Design review of the part built by this model. Coordinates are the model's own, in mm. Face numbers are marked on the shaded views. A direction names the side the tool comes from. Give positions to 0.01 mm unless a question says otherwise; leave off trailing zeros. Write each loop counter-clockwise with the first axis right and the second up, starting at its lowest first coordinate (ties: lowest second). Pieces come first, ordered by that corner, then holes. Notation, with made-up numbers: (69, -6) -> (80, -6) arc R13 cw to (80, 19) -> close; hole circle Ø10 at (-18.5, 25). An arc over 180 degrees is marked (long way). Answer as a JSON object with one key per item and string values.
Autodesk Fusion 360 part; units mm, degrees
sketch "Sketch1" plane through (0, 0, 0) normal (0, 0, 1) x (1, 0, 0)
  line L0 (21, -21) -> (-21, -21)
  line L1 (-21, -21) -> (-21, 21)
  line L2 (-21, 21) -> (21, 21)
  line L3 (21, 21) -> (21, -21)
  line L4 (21, -21) -> (-21, 21) construction
  line L5 (-21, -21) -> (21, 21) construction
  line L6 (0, 50) -> (0, -40)
  line L7 (-140, 50) -> (140, 50)
  line L8 (140, 50) -> (140, -130)
  line L9 (140, -130) -> (-140, -130)
  line L10 (-140, -130) -> (-140, 50)
  line L11 (-140, 50) -> (140, -130) construction
  line L12 (140, 50) -> (-140, -130) construction
  point P0 (0, -40)
  dimension "d1" = 42
  dimension "d2" = 42
  dimension "d14" = 280
extrude "Extrude4" add sketch "Sketch1" along normal blind 10
sketch "Sketch3" plane through (0, 0, 10) normal (0, 0, 1) x (-1, 0, 0)
  line L0 (21, -21) -> (-21, -21)
  line L1 (-21, -21) -> (-21, 21)
  line L2 (-21, 21) -> (21, 21)
  line L3 (21, 21) -> (21, -21)
  line L4 (140, 130) -> (-140, 130)
  line L5 (-140, 130) -> (-140, -50)
  line L6 (-140, -50) -> (140, -50)
  line L7 (140, -50) -> (140, 130)
  line L8 (-120, 120) -> (40, 120)
  line L9 (40, 120) -> (40, 35)
  line L10 (40, 35) -> (-120, 35)
  line L11 (-120, 35) -> (-120, 120)
  line L12 (70, 100) -> (126, 100)
  line L13 (126, 100) -> (126, 15)
  line L14 (126, 15) -> (70, 15)
  line L15 (70, 15) -> (70, 100)
  line L16 (-140, -50) -> (-135, -50)
  line L17 (-135, -50) -> (-135, 130)
  line L18 (-135, 130) -> (-140, 130)
  line L19 (-140, 130) -> (-140, -50)
  line L20 (-135, 130) -> (140, 130)
  line L21 (140, 130) -> (140, 125)
  line L22 (140, 125) -> (-135, 125)
  line L23 (-135, 125) -> (-135, 130)
  line L24 (140, 125) -> (135, 125)
  line L25 (135, 125) -> (135, -25)
  line L26 (135, -25) -> (140, -25)
  line L27 (140, -25) -> (140, 125)
  line L28 (135, -25) -> (25, -25)
  line L29 (25, -25) -> (25, -20)
  line L30 (25, -20) -> (135, -20)
  line L31 (135, -20) -> (135, -25)
  line L32 (25, -25) -> (-25, -25)
  line L33 (-25, -25) -> (-25, 25)
  line L34 (-25, 25) -> (25, 25)
  line L35 (25, 25) -> (25, -25)
  line L36 (25, -25) -> (-25, 25) construction
  line L37 (-25, -25) -> (25, 25) construction
  line L38 (-25, -25) -> (-135, -25)
  line L39 (-25, -21) -> (-135, -21)
  dimension "d17" = 160
  dimension "d18" = 85
  dimension "d19" = 56
  dimension "d20" = 85
  dimension "d24" = 5
  dimension "d25" = 5
  dimension "d26" = 5
  dimension "d29" = 50
  dimension "d30" = 50
extrude "Extrude6" add sketch "Sketch3" along normal blind 10 contours L4 L7 L17 L20 L21 L22 L23 L24 | L4 L5 L6 L16 L17 L18 L19 L23 | L7 L22 L24 L25 L26 L27 L31 | L25 L28 L29 L30 L31 L35
extrude "Extrude7" add sketch "Sketch3" along normal blind 10 contours L29 L32 L33 L34 L35
extrude "Extrude8" add sketch "Sketch3" along normal blind 10 contours L17 L33 L38 L39
sketch "Sketch4" plane through (0, 50, 0) normal (0, 1, 0) x (-1, 0, 0)
  line L0 (-140, 0) -> (140, 0)
  line L1 (140, 0) -> (140, 10)
  line L2 (140, 10) -> (-135, 10)
  line L3 (-135, 10) -> (-135, 20)
  line L4 (-135, 20) -> (-140, 20)
  line L5 (-140, 20) -> (-140, 0)
  line L6 (-140, 10) -> (-135, 10)
extrude "Extrude9" cut sketch "Sketch4" against normal blind 25 contours L3 L4 L5 L6
extrude "Extrude10" add 1 faces at (45, -128.3333, 20) along direction (0, 0, 1) blind 10
sketch "Sketch6" plane through (0, 0, 10) normal (0, 0, 1) x (-1, 0, 0)
  line L0 (-135, -21) -> (-25, -21)
  line L1 (-25, -21) -> (-25, 25)
  line L2 (-25, 25) -> (25, 25)
  line L3 (25, 25) -> (25, -20)
  line L4 (25, -20) -> (135, -20)
  line L5 (135, -20) -> (135, 125)
  line L6 (135, 125) -> (-135, 125)
  line L7 (-135, 125) -> (-135, -21)
  line L8 (0, 21) -> (0, 28)
  line L9 (0, 28) -> (0, 52)
  circle A0 centre (0, 28) radius 5
  circle A1 centre (0, 28) radius 7
  circle A2 centre (0, 52) radius 5
  circle A3 centre (0, 52) radius 7
  line L10 (7, 28) -> (7, 52)
  line L11 (-7, 28) -> (-7, 51)
  line L12 (5, 28) -> (5, 52)
  line L13 (-5, 28) -> (-5, 52)
  line L14 (-5, -50) -> (5, -50)
  line L15 (5, -50) -> (5, -25)
  line L16 (5, -25) -> (-5, -25)
  line L17 (-5, -25) -> (-5, -50)
  dimension "d39" = 7
  dimension "d40" = 10
  dimension "d41" = 10
  dimension "d42" = 14
extrude "Extrude11" cut sketch "Sketch6" against normal blind 20 contours L2 L8 L9 A0 | L2 L8 L9 A0 | L9 A0 A1 L13 | L9 A1 A3 L13 | L9 A0 A1 L12 | L9 A1 A3 L12 | L9 A2 A3 L13 | L9 A2 A3 L12 | A2
extrude "Extrude12" cut sketch "Sketch6" against normal blind 20 contours L14 L15 L16 L17
sketch "Sketch7" plane through (0, 21, 0) normal (0, -1, 0) x (1, 0, 0)
  line L0 (-21, 0) -> (21, 0)
  line L1 (21, 0) -> (21, 30)
  line L2 (21, 30) -> (-21, 30)
  line L3 (-21, 30) -> (-21, 0)
  line L4 (-21, 30) -> (21, 30)
  line L5 (21, 30) -> (21, 10)
  line L6 (21, 10) -> (-21, 10)
  line L7 (-21, 10) -> (-21, 30)
  dimension "d47" = 20
extrude "Extrude13" cut sketch "Sketch7" against normal blind 10 contours L1 L2 L3 L4 L5 L6 L7
extrude "Extrude14" cut 1 faces at (1.6667, 25, 3.3333) along direction (0, -1, 0) blind 5
extrude "Extrude15" add 2 faces at (50, 50, 3.3333) (-50, 50, 6.6667) along direction (0, 1, 0) blind 8
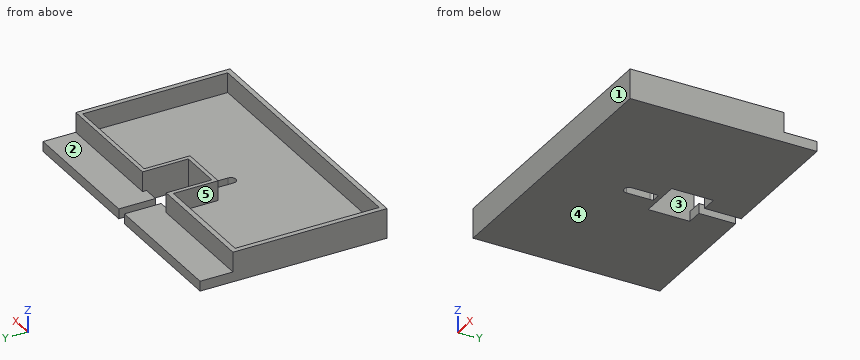
(1) For line 1 along X through (y, z) = (1.5, 19); line 2 along X through (y, z) = (-36.5, 22.25); line 3 along Y through (x, z) = (111.5, 17.5), list the stretches that pass through material, from the lowest coordinate up.
Here are the results:
{"line 1": "x = -140 to -135, -25 to -21, 21 to 25, 135 to 140", "line 2": "x = -140 to -135, 135 to 140", "line 3": "y = -130 to -125, 21 to 25"}
(2) We need section C-C, the plane x = -11.5. State the section outline as (y, z) points.
Here are the results:
{"outline": "(-130, 0) -> (-21, 0) -> (-21, 30) -> (-25, 30) -> (-25, 10) -> (-125, 10) -> (-125, 30) -> (-130, 30) -> close; (21, 0) -> (58, 0) -> (58, 10) -> (21, 10) -> close"}
(3) The part is to be moulded in two halves that separate along Y. For the marked faces 1, 2 and 3, say which applies: +Y half, -Y half, draft (parallel to the pull), parting line (faces both ways), or undercut.
Here are the results:
{"face 1": "-Y half", "face 2": "draft", "face 3": "undercut"}
(4) Clearance check with flat-ended pins moving along their axes: pin 1 (4 mm diameter, centred on x = -10, z = 21, fed in from +Y); pin 2 (10 mm diameter, centred on x = -95, z = 21, fed in from +Y); pin 3 (8 mm diameter, centred on x = -86.5, y = -49.5, fed in from +Z). State where each tip first meets the part, or that it passes through.
Here are the results:
{"pin 1": "stops at y = -21", "pin 2": "stops at y = 25", "pin 3": "stops at z = 10"}
(5) We need section A-A, the plane y = -40.5. State the section outline as (x, z) points, then the cut area to 3 significant figures.
Here are the results:
{"outline": "(-140, 0) -> (-5, 0) -> (-5, 10) -> (-135, 10) -> (-135, 30) -> (-140, 30) -> close; (5, 0) -> (140, 0) -> (140, 30) -> (135, 30) -> (135, 10) -> (5, 10) -> close", "area": "2,900 mm²"}
(6) We need section B-B, the plane z = 19.25. State the section outline as (x, y) points.
Here are the results:
{"outline": "(-140, -130) -> (140, -130) -> (140, 25) -> (21, 25) -> (21, -21) -> (-21, -21) -> (-21, 25) -> (-140, 25) -> close; hole (-135, -125) -> (135, -125) -> (135, 21) -> (25, 21) -> (25, -25) -> (-25, -25) -> (-25, 20) -> (-135, 20) -> close"}
(7) We need section D-D, the plane y = -87. State the section outline as (x, z) points.
Here are the results:
{"outline": "(-140, 0) -> (140, 0) -> (140, 30) -> (135, 30) -> (135, 10) -> (-135, 10) -> (-135, 30) -> (-140, 30) -> close"}
(8) For the marked faces 4 and 5, list the 3-axis set-ups (+Z, -Z, +X, -X, +Y, -Y) from which the entire face can be reached by the end or side of a thin tool; tool diameter is ignored.
Here are the results:
{"face 4": "-Z, +X, -X, +Y, -Y", "face 5": "+Z"}
